Here's how the part is built. I have some questions about the finished solid (model axes, mm). A direction names the side the tool comes from. Coordinates: 2 decimals unless noted, no trailing zeros. Order: outer loops, then holes, each group sorted by start corner. A loop starts at its lowest first (then second) coordinate and runs counter-clockwise, first axis right, second up.
```python
from build123d import *

# Parameters (mm, degrees)
F0_W      = 53
F0_H      = 26
F1_DEPTH  = 26
F2_W      = 11
F2_H      = 5
F3_DEPTH  = 7
F4_W      = 11
F4_H      = 5
F5_DEPTH  = 7
F7_DEPTH  = 53.001
F9_DEPTH  = 46.001
F12_DEPTH = 39
F14_W     = 17
F14_H     = 17
F15_DEPTH = 21.3027613393
F16_DEPTH = 39


with BuildPart() as f1:
    # F0 (on Front) → F1 (new body)
    with BuildSketch(Plane.XZ):
        Rectangle(F0_W, F0_H)
    extrude(amount=F1_DEPTH)

    # F2 (on face) → F3 (cut)
    with BuildSketch(Plane.YZ.offset(26.5)):
        with Locations((-5.5, 10.5)):
            Rectangle(F2_W, F2_H)
    extrude(amount=-F3_DEPTH, mode=Mode.SUBTRACT)

    # F4 (on face) → F5 (cut)
    with BuildSketch(Plane(origin=(-26.5, 0, 0), x_dir=(0, -1, 0), z_dir=(-1, 0, 0))):
        with Locations((5.5, 10.5)):
            Rectangle(F4_W, F4_H)
    extrude(amount=-F5_DEPTH, mode=Mode.SUBTRACT)

    # F6 (on face) → F7 (cut, through all)
    with BuildSketch(Plane.YZ.offset(26.5)):
        Polygon((-20.9308508784, 13), (-26, 13), (-26, 3.7), (-14, 3.7), (-11, 8), (-11, 13), align=None)
    extrude(amount=-F7_DEPTH, mode=Mode.SUBTRACT)

    # F8 (on face) → F9 (cut, through all)
    with BuildSketch(Plane.YZ.offset(19.5)):
        Polygon((-11, 13), (-11, 8), (-5, 13), align=None)
    extrude(amount=-F9_DEPTH, mode=Mode.SUBTRACT)

    # F11 (on offset) → F12 (cut)
    with BuildSketch(Plane(origin=(-19.5, 0, 0), x_dir=(0, -1, 0), z_dir=(-1, 0, 0))):
        Polygon((26, -13), (26, 3.7961313778), (11.3091202676, 7.9921598434), align=None)
    extrude(amount=-F12_DEPTH, mode=Mode.SUBTRACT)

    # F14 (on offset) → F15 (cut, through all)
    with BuildSketch(Plane(origin=(0, -11.3456357591, 7.9399819584), x_dir=(1, 0, 0), z_dir=(0, -0.8192985131, 0.5733672004))):
        with Locations((0, -10.1738724944)):
            Rectangle(F14_W, F14_H)
    extrude(amount=-F15_DEPTH, mode=Mode.SUBTRACT)

    # F11 (on offset) → F16 (cut)
    with BuildSketch(Plane(origin=(-19.5, 0, 0), x_dir=(0, -1, 0), z_dir=(-1, 0, 0))):
        Polygon((26, -13), (26, 3.7961313778), (11.3091202676, 7.9921598434), align=None)
    extrude(amount=-F16_DEPTH, mode=Mode.SUBTRACT)


solid = f1.part
```
Q1. For faces 1 (the flat face through (-0.119, -6.134, 2.25)), 2 (the flat face through (-0.12, -18.08, -10.14)), 3 (the flat face through (-23, -20, 3.7)), which set-ups out of +Z, -Z, +X, -X, +Y, -Y let a thin tool reach every point of the face, with its end or its side?
Q2. Will these pins go through, and if not, where does the flat tip stop? pin 1 (2 mm diameter, centred on x = 13.5, z = 2.5, fed in from -Y); pin 2 (2.5 mm diameter, centred on y = -4.5, z = 9.5, fed in from -X); pin 3 (3.5 mm diameter, centred on x = 23.5, y = -5, fed in from +Z).
Q3. If we section it at D-D on z = 2: Write out the boundary of the cut face in (x, y).
Q4. If we section it at A-A on z = -4.75: Write out the boundary of the cut face in (x, y).
Q5. I need wall thicknesses on L1, parallel to X at y = -8, z = -9.5; L2, parallel to X at y = -23.75, z = 2.25; L3, parallel to Z at x = 23, y = -20. Which ranges of each line are inside material? Lowest first, please.
Q6. We'd pull the mould along X, two halves only. Please class faces 4 (the flat face through (-19.5, -23, -1)), 5 (the flat face through (-26.5, -13, -3)), 6 (the flat face through (-23, -26, -5)): pulls with the +X half, pulls with the -X half, needs draft (parallel to the pull), parting line crosses it, or undercut.
Q7. If we section it at C-C on y = -8.5: Write out the boundary of the cut face in (x, z).
Q8. If we section it at B-B on x = -12: Write out the boundary of the cut face in (y, z).
Reply:
1. face 1: -Z, -Y
1. face 2: +Z, +Y
1. face 3: +Z, +X, -X, -Y
2. pin 1: stops at y = -15.85
2. pin 2: stops at x = -19.5
2. pin 3: stops at z = 8
3. outline: (-26.5, -26) - (-19.5, -26) - (-19.5, -15.5) - (-8.5, -15.5) - (-8.5, -5.78) - (8.5, -5.78) - (8.5, -15.5) - (19.5, -15.5) - (19.5, -26) - (26.5, -26) - (26.5, 0) - (-26.5, 0) - close
4. outline: (-26.5, -26) - (-19.5, -26) - (-19.5, -20.23) - (-8.5, -20.23) - (-8.5, 0) - (-26.5, 0) - close; (8.5, -20.23) - (19.5, -20.23) - (19.5, -26) - (26.5, -26) - (26.5, 0) - (8.5, 0) - close
5. L1: x = -26.5 to -8.5, 8.5 to 26.5
5. L2: x = -26.5 to -19.5, 19.5 to 26.5
5. L3: z = -13 to 3.7
6. face 4: undercut
6. face 5: pulls with the -X half
6. face 6: needs draft
7. outline: (-26.5, -13) - (-8.5, -13) - (-8.5, 3.91) - (8.5, 3.91) - (8.5, -13) - (26.5, -13) - (26.5, 8) - (19.5, 8) - (19.5, 10.08) - (-19.5, 10.08) - (-19.5, 8) - (-26.5, 8) - close
8. outline: (-26, -13) - (0, -13) - (0, 13) - (-5, 13) - (-11, 8) - (-14, 3.7) - (-14.31, 3.7) - close
